from build123d import *

# Parameters (mm, degrees)
SKETCH1_W           = 60
SKETCH1_H           = 60
SKETCH1_R           = 2
BOSS_EXTRUDE1_DEPTH = 48


with BuildPart() as part:
    # Sketch1 → Boss-Extrude1 (new body)
    with BuildSketch(Plane(origin=(0, 0, 0), x_dir=(1, 0, 0), z_dir=(0, 1, 0))):
        Rectangle(SKETCH1_W, SKETCH1_H)
        with Locations((-25, 25)):
            Circle(SKETCH1_R, mode=Mode.SUBTRACT)
        with Locations((25, 25)):
            Circle(SKETCH1_R, mode=Mode.SUBTRACT)
        with Locations((25, -25)):
            Circle(SKETCH1_R, mode=Mode.SUBTRACT)
        with Locations((-25, -25)):
            Circle(SKETCH1_R, mode=Mode.SUBTRACT)
    extrude(amount=BOSS_EXTRUDE1_DEPTH)

    # Sketch3 → Revolve1 (revolve)
    with BuildSketch(Plane.XY):
        Polygon((0, 48), (18, 48), (18, 49.5), (4, 49.5), (4, 57.5), (0, 57.5), align=None)
    revolve(axis=Axis((0, 57.5, 0), (0, -1, 0)))


solid = part.part
Geometry: final body of the model. Coordinates: model frame, mm. A direction names the side the tool comes from. Round coordinates to 2 decimals unless told otherwise and drop trailing zeros. Order: outer loops, then holes, each group sorted by start corner. A loop starts at its lowest first (then second) coordinate and runs counter-clockwise, first axis right, second up. Notation, with made-up numbers: (27, 85) -> (77, 85) arc R19 ccw to (77, 117) -> close; hole circle Ø8 at (76, 59.5). An arc over 180 degrees is marked (long way). Put each result on its own line as item: value. Start each with the question number.
Q1. Section D-D on x = 1.5. Return the cut outline in (y, z).
Q2. Line query: probe 1 along X at (y, z) = (32, -25); probe 2 along Z at (x, y) = (24, 11.5). Output: solid intervals per line, ascending.
Q3. Reachability of faces 5 (the cylindrical face through (-2.343, 48.76, 17.847)), 6 (the flat face through (0, 57.5, 0)) from +Z, -Z, +X, -X, +Y, -Y: full face, straight path, thin tool, end or side. Return the list, or none.
Q4. Section B-B on z = 0. Return the cut outline in (x, y).
Q5. Pull-direction query (Z, two-part tool) for faces 1 (the cylindrical face through (23.4, 23.7, 26.2)), 2 (the flat face through (-4.3, 49.5, 0.3)), 3 (the flat face through (0, 24, 30)), 4 (the flat face through (0, 24, -30)); classes: +Z half, -Z half, draft (parallel to the pull), parting line (faces both ways), or undercut.
Q6. Section A-A on x = -25. Return the cut outline in (y, z).
Q7. Section C-C on z = -25. Return the cut outline in (x, y).
Q8. First-contact query: pin 1 (8 mm diameter, centred on x = -5, z = -17, fed in from +Y). Flat tip, straight axial feed; report the tip coordinate or a pass-through.
Ans:
1. outline: (0, -30) -> (48, -30) -> (48, -17.94) -> (49.5, -17.94) -> (49.5, -3.71) -> (57.5, -3.71) -> (57.5, 3.71) -> (49.5, 3.71) -> (49.5, 17.94) -> (48, 17.94) -> (48, 30) -> (0, 30) -> close
2. probe 1: x = -30 to -27, -23 to 23, 27 to 30
2. probe 2: z = -30 to -26.73, -23.27 to 23.27, 26.73 to 30
3. face 5: +Y
3. face 6: +Z, -Z, +X, -X, +Y
4. outline: (-30, 0) -> (30, 0) -> (30, 48) -> (18, 48) -> (18, 49.5) -> (4, 49.5) -> (4, 57.5) -> (-4, 57.5) -> (-4, 49.5) -> (-18, 49.5) -> (-18, 48) -> (-30, 48) -> close
5. face 1: undercut
5. face 2: draft
5. face 3: +Z half
5. face 4: -Z half
6. outline: (0, -30) -> (48, -30) -> (48, -27) -> (0, -27) -> close; (0, -23) -> (48, -23) -> (48, 23) -> (0, 23) -> close; (0, 27) -> (48, 27) -> (48, 30) -> (0, 30) -> close
7. outline: (-30, 0) -> (-27, 0) -> (-27, 48) -> (-30, 48) -> close; (-23, 0) -> (23, 0) -> (23, 48) -> (-23, 48) -> close; (27, 0) -> (30, 0) -> (30, 48) -> (27, 48) -> close
8. pin 1: stops at y = 49.5
